from build123d import *

# Parameters (mm, degrees)
SKETCH1_W           = 120
SKETCH1_H           = 40
SKETCH1_W_2         = 30.073092916
SKETCH1_H_2         = 5
SKETCH1_W_3         = 30
BOSS_EXTRUDE1_DEPTH = 5


with BuildPart() as part:
    # Sketch1 → Boss-Extrude1 (new body)
    with BuildSketch(Plane.XY):
        Rectangle(SKETCH1_W, SKETCH1_H)
        with Locations((34.956464204, 12.5)):
            Rectangle(SKETCH1_W_2, SKETCH1_H_2, mode=Mode.SUBTRACT)
        with Locations((-35, 12.5)):
            Rectangle(SKETCH1_W_3, SKETCH1_H_2, mode=Mode.SUBTRACT)
        with Locations((-35, -12.5)):
            Rectangle(SKETCH1_W_3, SKETCH1_H_2, mode=Mode.SUBTRACT)
        with Locations((35, -12.5)):
            Rectangle(SKETCH1_W_3, SKETCH1_H_2, mode=Mode.SUBTRACT)
        with Locations((-35, -22.5)):
            Rectangle(SKETCH1_W_3, SKETCH1_H_2)
        with Locations((35, -22.5)):
            Rectangle(SKETCH1_W_3, SKETCH1_H_2)
        with Locations((35, 22.5)):
            Rectangle(SKETCH1_W_3, SKETCH1_H_2)
        with Locations((-35, 22.5)):
            Rectangle(SKETCH1_W_3, SKETCH1_H_2)
    extrude(amount=BOSS_EXTRUDE1_DEPTH)


solid = part.part
Part model, mm, in its own coordinate system. A direction names the side the tool comes from. Coordinates: 2 decimals unless noted, no trailing zeros. Loops run counter-clockwise (first coordinate to the right, second up) from the corner with the lowest first, then second, coordinate; pieces in that order, holes last. Notation, with made-up numbers: (-11.75, -28) -> (-4.75, -28) arc R18 ccw to (-4.75, -21) -> close; hole circle Ø4 at (87, 37). An arc over 180 degrees is marked (long way). Use a Markdown table: item, result. Add a question column.
Item 1: Probe probe 1 along X at (y, z) = (-14, 0.3); probe 2 along Y at (x, z) = (27, 0.55); probe 3 along X at (y, z) = (-22, 0.5). List the from-to ranges inside material, lowest first.
Item 2: Band-saw the part on C-C on z = 3.25. Give the number of separate pieces and of enclosed holes in the cut face, plus the area to 3 significant figures.
Item 3: Band-saw the part on D-D on x = 3.5. Write the cut outline in (y, z), plus the area to 3 significant figures.
Item 4: Band-saw the part on B-B on x = 36. Write the cut outline in (y, z), plus the area to 3 significant figures.
Item 5: Which spindle directions (+Z, -Z, +X, -X, +Y, -Y) get a long thin tool onto all of the face, cutting with end or side? Do faces 4 (the flat face through (20, 22, 2)), 5 (the flat face through (50, -23, 2)), 6 (the flat face through (20, -13, 2)), 7 (the flat face through (20, -23, 2)). Say none if no direction does.
Item 6: Band-saw the part on A-A on y = 13. Write the cut outline in (x, z).
Item 7: Flat gauge pins, fed straight in: P1, Ø2.5, axis at y = -22, z = 2.5, coming from the +X side; P2, Ø2.5, axis at x = 55.5, z = 2, coming from the -Y side. Where does each tip first touch, or does it go through?
Item 8: Pull direction X, two halves, no side cores. Call faces 1 (the flat face through (60, 0, 2)), 2 (the flat face through (50, -13, 2)), 3 (the flat face through (55, -20, 2)): +X half, -X half, draft (parallel to the pull), parting line (faces both ways), or undercut.
Geometry says:
| question | item | result |
|---|---|---|
| 1 | probe 1 | -60 to -50, -20 to 20, 50 to 60 |
| 1 | probe 2 | -25 to -15, -10 to 10, 15 to 25 |
| 1 | probe 3 | -50 to -20, 20 to 50 |
| 2 | separate pieces | 1 |
| 2 | enclosed holes | 4 |
| 2 | area | 4,800 mm² |
| 3 | outline | (-20, 0) -> (20, 0) -> (20, 5) -> (-20, 5) -> close |
| 3 | area | 200 mm² |
| 4 | outline | (-25, 0) -> (-15, 0) -> (-15, 5) -> (-25, 5) -> close; (-10, 0) -> (10, 0) -> (10, 5) -> (-10, 5) -> close; (15, 0) -> (25, 0) -> (25, 5) -> (15, 5) -> close |
| 4 | area | 200 mm² |
| 5 | face 4 | +Z, -Z, +Y |
| 5 | face 5 | +Z, -Z, +X, -Y |
| 5 | face 6 | +Z, -Z |
| 5 | face 7 | +Z, -Z, -Y |
| 6 | outline | (-60, 0) -> (-50, 0) -> (-50, 5) -> (-60, 5) -> close; (-20, 0) -> (19.92, 0) -> (19.92, 5) -> (-20, 5) -> close; (49.99, 0) -> (60, 0) -> (60, 5) -> (49.99, 5) -> close |
| 7 | P1 | x = 50 |
| 7 | P2 | y = -20 |
| 8 | face 1 | +X half |
| 8 | face 2 | undercut |
| 8 | face 3 | draft |
